The listing builds one solid part. Answer for the finished solid, in the listing's coordinates (mm). Round coordinates to 2 decimals unless told otherwise and drop trailing zeros. Write each loop counter-clockwise with the first axis right and the second up, starting at its lowest first coordinate (ties: lowest second). Pieces come first, ordered by that corner, then holes.
Item 1: This flat-tipped pin is pushed along its axis until it touches: pin 1 (4 mm diameter, centred on x = -21.5, y = -4.5, fed in from -Z). Where does it stop, or does it pass through?
Item 2: Find section A-A on x = 28.5. Give the vertices of the cut face in (y, z).
Item 3: Find section B-B on y = 1.5. Give the vertices of the cut face in (x, z).
Item 4: Find the intervals of material crossed by probe 1 along X at (y, z) = (3.25, 5); probe 2 along Y at (x, z) = (8, -5.5), in increasing order.
```python
from build123d import *

# Parameters (mm, degrees)
BOSS_EXTRUDE1_DEPTH = 59.5
SKETCH5_W           = 1.1684
SKETCH5_H           = 8.939323218


with BuildPart() as part:
    # Sketch2 → Boss-Extrude1 (new, symmetric)
    with BuildSketch(Plane(origin=(0, 0, 0), x_dir=(0, 0, -1), z_dir=(1, 0, 0))):
        Polygon((7.332348419, 0), (3.666174209, 6.35), (-3.666174209, 6.35), (-7.332348419, 0), (-3.666174209, -6.35), (3.666174209, -6.35), align=None)
    extrude(amount=BOSS_EXTRUDE1_DEPTH, both=True)

    # Sketch5 → Cut-Revolve1 (revolve, cut)
    with BuildSketch(Plane.XY, mode=Mode.PRIVATE) as cut_revolve1_sk:
        with Locations((13.0658, 9.498861609)):
            Rectangle(SKETCH5_W, SKETCH5_H)
        with Locations((-6.7658, 9.498861609)):
            Rectangle(SKETCH5_W, SKETCH5_H)
    revolve(cut_revolve1_sk.sketch.rotate(Axis((0, 0, 0), (1, 0, 0)), 90), axis=Axis((0, 0, 0), (1, 0, 0)), mode=Mode.SUBTRACT)


solid = part.part
```
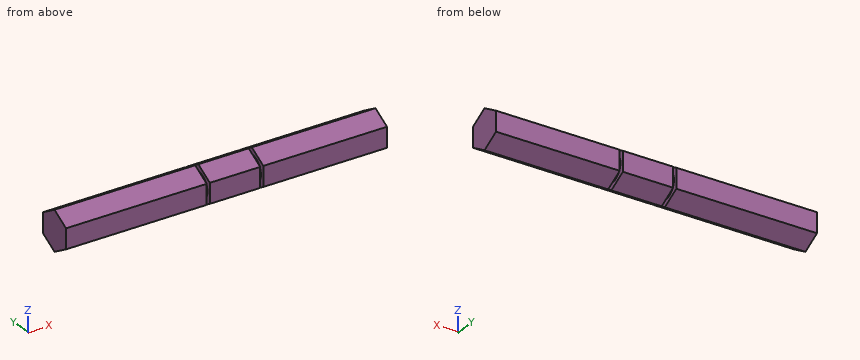
Check values:
1. pin 1: stops at z = -5.89
2. outline: (-6.35, -3.67) - (0, -7.33) - (6.35, -3.67) - (6.35, 3.67) - (0, 7.33) - (-6.35, 3.67) - close
3. outline: (-59.5, -6.47) - (-7.35, -6.47) - (-7.35, -4.8) - (-6.18, -4.8) - (-6.18, -6.47) - (12.48, -6.47) - (12.48, -4.8) - (13.65, -4.8) - (13.65, -6.47) - (59.5, -6.47) - (59.5, 6.47) - (13.65, 6.47) - (13.65, 4.8) - (12.48, 4.8) - (12.48, 6.47) - (-6.18, 6.47) - (-6.18, 4.8) - (-7.35, 4.8) - (-7.35, 6.47) - (-59.5, 6.47) - close
4. probe 1: x = -59.5 to -7.35, -6.18 to 12.48, 13.65 to 59.5
4. probe 2: y = -3.17 to 3.17
